Input: part model. Units: mm. Frame: model coordinates. A direction names the side the tool comes from. Coordinates: 2 decimals unless noted, no trailing zeros. Loops run counter-clockwise (first coordinate to the right, second up) from the corner with the lowest first, then second, coordinate; pieces in that order, holes last. Notation, with made-up numbers: (-39.75, 6.25) -> (-33.75, 6.25) arc R17 cw to (-33.75, 23.25) -> close; hole circle Ø3 at (55, -26). An arc over 180 degrees is marked (long way). Put each result on its own line as item: value. Start each with the question number.
1) Cut plane D-D (z = 170). Return the cut outline in (x, y).
2) Material intervals for L1, parallel to X at y = -10, z = 95; L2, parallel to X at y = -6, z = 95; L3, parallel to Y at x = -65.5, z = 164, sorted ascending.
3) Cut plane C-C (z = 43). Return the cut outline in (x, y).
4) Pull-direction query (X, two-part tool) for faces 1 (the cylindrical face through (-525.515, 38.967, 93.916)), 2 (the flat face through (-95, -9, 120.25)), 3 (the flat face through (-245, -19, 94)); classes: pulls with the +X half, pulls with the -X half, needs draft (parallel to the pull), parting line crosses it, or undercut.
5) Cut plane A-A (x = -74). Return the cut outline in (y, z), plus the area to 3 significant figures.
6) Contact query for flat-ended pins moving along their axis: P1, Ø2, axis at y = 283.5, z = 166, coming from the +X side; P2, Ø1.5, axis at y = 322.5, z = 123, coming from the -X side; P3, Ø12, axis at y = 219, z = 127, coming from the -X side. Output: stop coordinate, or through.
7) Cut plane B-B (z = 95.25). Return the cut outline in (x, y), plus the area to 3 significant figures.
8) Set-up query: faces 4 (the flat face through (-94, -9, 70.25)), 5 (the flat face through (-410, 176, 190.5)). Return all of +Z, -Z, +X, -X, +Y, -Y with unobstructed straight access to the full face (end or side cutting, diameter ignored); none if empty.
from build123d import *

# Parameters (mm, degrees)
F1_DEPTH = 190.5
F2_R     = 50
F3_R     = 15
F4_DEPTH = 101.6
F5_R     = 25
F6_DEPTH = 101.6


with BuildPart() as f1:
    # F0 (on Top) → F1 (new body)
    with BuildSketch(Plane.XY):
        with BuildLine():
            Line((7.8734308481, 0), (-480.600476265, 0))
            ThreePointArc((-480.600476265, 0), (-507.3725322107, 39.5160081985), (-492.1265691519, 84.7467333078))
            Line((-492.1265691519, 84.7467333078), (-185.7195747427, 391.1537277171))
            Line((-185.7195747427, 391.1537277171), (-199.1546035852, 404.5887565596))
            Line((-199.1546035852, 404.5887565596), (-503.0509646748, 100.69239547))
            ThreePointArc((-503.0509646748, 100.69239547), (-525.4247574788, 38.0082411155), (-491.0743534565, -19))
            Line((-491.0743534565, -19), (7.8734308481, -19))
            Line((7.8734308481, -19), (7.8734308481, 0))
        make_face()
    extrude(amount=F1_DEPTH)

    # F2
    f2_edges = [f1.edges().sort_by_distance(p)[0] for p in [
        (-192.437089, 397.871242, 190.5),
        (-192.437089, 397.871242, 0),
        (7.873431, -9.5, 190.5),
        (7.873431, -9.5, 0),
    ]]
    fillet(f2_edges, radius=F2_R)

    # F3 (on face) → F4 (cut)
    with BuildSketch(Plane(origin=(-301.8716800724, 301.8716800724, 0), x_dir=(-0.7071067812, -0.7071067812, 0), z_dir=(-0.7071067812, 0.7071067812, 0))):
        with Locations((-70.2638826555, 145.5)):
            Circle(F3_R)
        with Locations((-70.2638826555, 50)):
            Circle(F3_R)
    extrude(amount=-F4_DEPTH, mode=Mode.SUBTRACT)

    # F5 (on face) → F6 (cut)
    with BuildSketch(Plane(origin=(0, 0, 0), x_dir=(-1, 0, 0), z_dir=(0, 1, 0))):
        with Locations((312.1265691519, 95.25)):
            Circle(F5_R)
        with BuildLine():
            Line((152.1265691519, 120.25), (37.1265691519, 120.25))
            ThreePointArc((37.1265691519, 120.25), (12.1265691519, 95.25), (37.1265691519, 70.25))
            Line((37.1265691519, 70.25), (152.1265691519, 70.25))
            ThreePointArc((152.1265691519, 70.25), (177.1265691519, 95.25), (152.1265691519, 120.25))
        make_face()
    extrude(amount=-F6_DEPTH, mode=Mode.SUBTRACT)


solid = f1.part
Results found:
1. outline: (-503.05, 100.69) arc R77.71 ccw to (-491.07, -19) -> (-1.76, -19) -> (-1.76, 0) -> (-480.6, 0) arc R53.73 cw to (-492.13, 84.75) -> (-192.53, 384.34) -> (-205.96, 397.78) -> close
2. L1: x = -502.24 to -337.13, -287.13 to -177.13, -12.13 to 7.87
2. L2: x = -506.08 to -337.13, -287.13 to -177.13, -12.13 to 7.87
2. L3: y = -19 to 0
3. outline: (-503.05, 100.69) arc R77.71 ccw to (-491.07, -19) -> (7.38, -19) -> (7.38, 0) -> (-480.6, 0) arc R53.73 cw to (-492.13, 84.75) -> (-248.13, 328.74) -> (-261.57, 342.17) -> close; (-242.81, 360.94) -> (-229.37, 347.5) -> (-186.07, 390.81) -> (-199.5, 404.24) -> close
4. face 1: pulls with the -X half
4. face 2: undercut
4. face 3: needs draft
5. outline: (-19, 0) -> (0, 0) -> (0, 70.25) -> (-19, 70.25) -> close; (-19, 120.25) -> (0, 120.25) -> (0, 190.5) -> (-19, 190.5) -> close
5. area: 2,670 mm2
6. P1: stops at x = -292.37
6. P2: stops at x = -281.99
6. P3: stops at x = -390.74
7. outline: (-503.05, 100.69) arc R77.71 ccw to (-491.07, -19) -> (-337.13, -19) -> (-337.13, 0) -> (-480.6, 0) arc R53.73 cw to (-492.13, 84.75) -> (-185.72, 391.15) -> (-199.15, 404.59) -> close; (-287.13, -19) -> (-177.13, -19) -> (-177.13, 0) -> (-287.13, 0) -> close; (-12.13, -19) -> (7.87, -19) -> (7.87, 0) -> (-12.13, 0) -> close
7. area: 15,700 mm2
8. face 4: +Y, -Y
8. face 5: +Z, +X, -X, +Y, -Y
